```python
from build123d import *

# Parameters (mm, degrees)
SKETCH_1_R          = 1.7
EXTRUDE_1_DEPTH     = 5.8
SKETCH_2_W          = 5.8
SKETCH_2_H          = 48.387548751
CUT_EXTRUDE_1_DEPTH = 279.6
FILLET_1_R          = 6


with BuildPart() as part:
    # 草图1 → 凸台-拉伸1 (new body, symmetric)
    with BuildSketch(Plane.XY):
        with BuildLine():
            Line((-181.16239443, 23.937096774), (-179.662464671, -131.048387097))
            ThreePointArc((-179.662464671, -131.048387097), (-174.662698808, -136), (-169.662932944, -131.048387097))
            Line((-169.662932944, -131.048387097), (-168.163003185, 23.937096774))
            ThreePointArc((-168.163003185, 23.937096774), (-168.494379467, 26.049838166), (-169.49346521, 27.940688267))
            ThreePointArc((-169.49346521, 27.940688267), (-177.025820297, 49.382777319), (-170.5438245, 71.165414592))
            ThreePointArc((-170.5438245, 71.165414592), (-173.107050096, 78.751837233), (-179.660448301, 74.15))
            Line((-179.660448301, 74.15), (-181.159773149, 24.195))
            ThreePointArc((-181.159773149, 24.195), (-181.162363098, 24.06606139), (-181.16239443, 23.937096774))
        make_face()
        with Locations((-174.662698808, 24)):
            Circle(SKETCH_1_R, mode=Mode.SUBTRACT)
        with Locations((-174.662698808, -131)):
            Circle(SKETCH_1_R, mode=Mode.SUBTRACT)
        with Locations((-174.662698808, 74)):
            Circle(SKETCH_1_R, mode=Mode.SUBTRACT)
    extrude(amount=EXTRUDE_1_DEPTH, both=True)

    # 草图2 → 切除-拉伸1 (cut)
    with BuildSketch(Plane(origin=(0, 0, 0), x_dir=(0, 0, -1), z_dir=(1, 0, 0))):
        with Locations((2.9, 54.806225625)):
            Rectangle(SKETCH_2_W, SKETCH_2_H)
    extrude(amount=-CUT_EXTRUDE_1_DEPTH, mode=Mode.SUBTRACT)

    # 圆角1
    fillet_1_edges = [part.edges().sort_by_distance(p)[0] for p in [
        (-180.967162918, 30.612451249, -2.9),
        (-171.349640462, 30.612451249, -2.9),
    ]]
    fillet(fillet_1_edges, radius=FILLET_1_R)


solid = part.part
```
The model under review builds one solid part; all positions refer to its coordinate system, in mm. A direction names the side the tool comes from. Give positions to 0.01 mm unless a question says otherwise; leave off trailing zeros. Write each loop counter-clockwise with the first axis right and the second up, starting at its lowest first coordinate (ties: lowest second). Pieces come first, ordered by that corner, then holes.
(1) Tool access review of faces 1 (the cylindrical face through (-179.37, 28.87, -2.86)), 2 (the cylindrical face through (-172.98, 78.71, 2.94)), 3 (the cylindrical face through (-171.78, 29.96, -2.86)): name each direction out of +Z, -Z, +X, -X, +Y, -Y from which nothing blocks a thin tool from reaching the whole face with its end or side.
(2) For P1, Ø3, axis at y = -84, z = -0.5, coming from the -X side; P2, Ø5, axis at x = -179, z = 3.5, coming from the +Y side; P3, Ø6, axis at y = -111, z = 0, coming from the +X side, all flat-tipped, find the tip position at first contact; note any pin that passes through.
(3) To check wall thickness, follow L1, parallel to X at y = 74, z = 2.7; L2, parallel to Y at x = -170.5, z = 0.5; L3, parallel to Z at x = -180, y = 34. State the ranges of each line that lie inside material, in increasing order.
(4) Consider section A-A, the plane z = 3.25. Give the boundary of the cut face in (x, y) (3 decimals), and give its area (3 significant figures).
(5) Consider section C-C, the plane y = 57.5. Give the boundary of the cut face in (x, z).
(6) Consider section B-B, the plane y = -20. Give the boundary of the cut face in (x, z), and give its area (3 significant figures).
Returned:
1. face 1: -Z, -X, +Y
1. face 2: +Z, -Z
1. face 3: -Z, +X, +Y
2. P1: stops at x = -180.13
2. P2: stops at y = 78.65
2. P3: stops at x = -169.44
3. L1: x = -179.66 to -176.36, -172.96 to -169.66
3. L2: y = -133.77 to 29.33, 71.23 to 76.77
3. L3: z = 0 to 5.8
4. outline: (-181.162, 23.937) - (-179.662, -131.048) arc R5 ccw to (-169.663, -131.048) - (-168.163, 23.937) arc R6.5 ccw to (-169.493, 27.941) arc R36.844 cw to (-170.544, 71.165) arc R5 ccw (long way) to (-179.66, 74.15) - (-181.16, 24.195) arc R6.5 ccw to start; hole circle Ø3.4 at (-174.663, -131); hole circle Ø3.4 at (-174.663, 24); hole circle Ø3.4 at (-174.663, 74)
4. area: 2,150 mm2
5. outline: (-180.16, 0) - (-176.32, 0) - (-176.32, 5.8) - (-180.16, 5.8) - close
6. outline: (-180.74, -5.8) - (-168.59, -5.8) - (-168.59, 5.8) - (-180.74, 5.8) - close
6. area: 141 mm2
